Here's the drawing with two shaded views (mm, measured from the low corner). I have some questions. A direction names the side the tool comes from. Coordinates: 2 decimals unless noted, no trailing zeros. Loops run counter-clockwise (first coordinate to the right, second up) from the corner with the lowest first, then second, coordinate; pieces in that order, holes last. Notation, with made-up numbers: (49, 68.5) - (108, 68.5) arc R18 ccw to (108, 103.5) - close; hole circle Ø8 at (-21, 4.5). An arc over 180 degrees is marked (long way). Use a Markdown table: item, result.
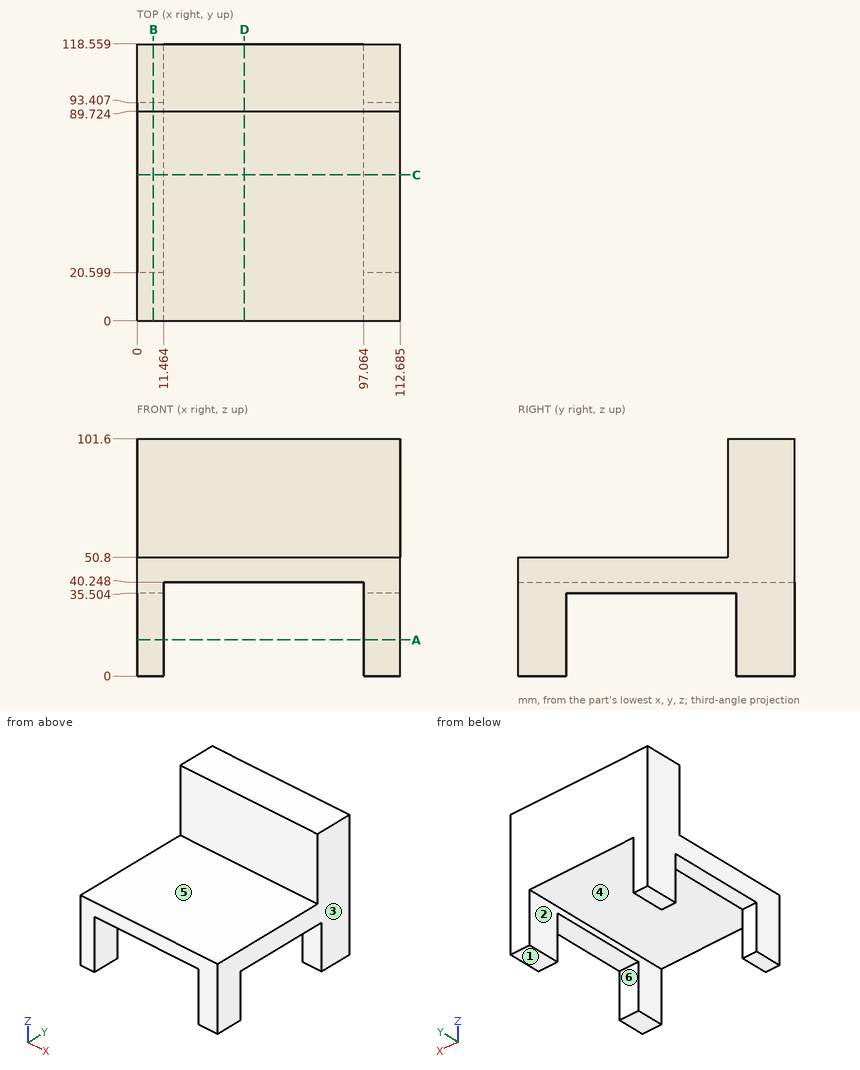
Q1. Will these pins go through, and if not, where does the flat tip stop? P1, Ø17, axis at x = 107.5, y = 45.5, coming from the -Z side; P2, Ø4, axis at x = 56, z = 86, coming from the -Y side; P3, Ø12, axis at x = 37, y = 24.5, coming from the +Z side.
Check values:
| item | result |
|---|---|
| P1 | z = 35.5 |
| P2 | y = 89.72 |
| P3 | z = 50.8 |
Q2. I want a section at B-B, the plane x = 7. Write out the boundary of the cut face in (y, z) (1 decimal).
Check values:
| item | result |
|---|---|
| outline | (0, 0) - (20.6, 0) - (20.6, 35.5) - (93.4, 35.5) - (93.4, 0) - (118.6, 0) - (118.6, 101.6) - (89.7, 101.6) - (89.7, 50.8) - (0, 50.8) - close |
Q3. I want a section at A-A, the plane z = 15.5. Write out the boundary of the cut face in (x, y) (1 decimal).
Check values:
| item | result |
|---|---|
| outline | (0, 0) - (11.5, 0) - (11.5, 20.6) - (0, 20.6) - close; (0, 93.4) - (11.5, 93.4) - (11.5, 118.6) - (0, 118.6) - close; (97.1, 0) - (112.7, 0) - (112.7, 20.6) - (97.1, 20.6) - close; (97.1, 93.4) - (112.7, 93.4) - (112.7, 118.6) - (97.1, 118.6) - close |
Q4. I want a section at C-C, the plane y = 62.5. Write out the boundary of the cut face in (x, z) (1 decimal), then the cut area to 3 significant figures.
Check values:
| item | result |
|---|---|
| outline | (0, 35.5) - (11.5, 35.5) - (11.5, 40.2) - (97.1, 40.2) - (97.1, 35.5) - (112.7, 35.5) - (112.7, 50.8) - (0, 50.8) - close |
| area | 1,320 mm^2 |
Q5. I want a section at D-D, the plane x = 46. Write out the boundary of the cut face in (y, z).
Check values:
| item | result |
|---|---|
| outline | (0, 40.25) - (118.56, 40.25) - (118.56, 101.6) - (89.72, 101.6) - (89.72, 50.8) - (0, 50.8) - close |
Q6. Which directions (+Z, -Z, +X, -X, +Y, -Y) give clear straight access to the entire face, cutting with the end or side of a thin tool? Please do the marked faces 4, 5 and 6.
Check values:
| item | result |
|---|---|
| face 4 | -Z, +Y, -Y |
| face 5 | +Z, +X, -X, -Y |
| face 6 | -Z, +X, -X |
Q7. Please list where these lines run through material, in increasing order: L1, parallel to X at y = 94, z = 24 (1 decimal); L2, parallel to Y at x = 99.5, z = 17; L3, parallel to Y at x = 102, z = 62.5. Write a range as from..to.
Check values:
| item | result |
|---|---|
| L1 | 0..11.5, 97.1..112.7 |
| L2 | 0..20.6, 93.41..118.56 |
| L3 | 89.72..118.56 |
Q8. If we mould it in two halves opening along X, with no side actions, what happens to the marked faces 1, 2 and 3? For each: pulls with the +X half, pulls with the -X half, needs draft (parallel to the pull), parting line crosses it, or undercut.
Check values:
| item | result |
|---|---|
| face 1 | needs draft |
| face 2 | undercut |
| face 3 | pulls with the +X half |
